Autodesk Inventor part; units mm, degrees
ref_plane "YZ Plane" through (0, 0, 0) normal (1, 0, 0) x (0, 1, 0)
ref_plane "XZ Plane" through (0, 0, 0) normal (0, 1, 0) x (-1, 0, 0)
ref_plane "XY Plane" through (0, 0, 0) normal (0, 0, 1) x (1, 0, 0)
sketch "草圖1" plane through (0, 0, 0) normal (0, 1, 0) x (-1, 0, 0)
  circle A0 centre (0, 0) radius 46.75
  circle A1 centre (0, 0) radius 44.75
  dimension "d0" = 93.5
  dimension "d1" = 2
extrude "擠出1" add sketch "草圖1" along normal blind 10
sketch "草圖2" plane through (0, 10, 0) normal (0, 1, 0) x (1, 0, 0)
  circle A0 centre (0, 0) radius 50
  dimension "d4" = 100
extrude "擠出2" add sketch "草圖2" along normal blind 2
sketch "草圖4" plane through (0, 0, 0) normal (1, 0, 0) x (0, 1, 0)
  line L0 (12, -50) -> (12, 50)
  line L1 (12, -25.0248) -> (30.0379, -25.0248)
  line L2 (30.0379, -25.0248) -> (30.0379, 11.7448)
  line L3 (30.0379, 11.7448) -> (12, 11.7448)
  line L4 (12, 11.7448) -> (12, -25.0248)
  line L5 (30.0379, -25.0248) -> (72.4644, 17.4017)
  line L6 (72.4644, 17.4017) -> (54.0796, 35.7864)
  line L7 (54.0796, 35.7864) -> (11.6532, -6.64)
  line L8 (11.6532, -6.64) -> (30.0379, -25.0248)
  point P0 (0, 0)
  dimension "d12" = 45
  dimension "d13" = 26
  dimension "d14" = 60
extrude "擠出4" add sketch "草圖4" along normal blind 5
fillet "圓角1" radius 10 1 edges at (2.5, 30.0379, 11.7448)
fillet "圓角2" radius 10 1 edges at (2.5, 30.0379, -25.0248)
sketch "草圖5" plane through (5, 0, 0) normal (1, 0, 0) x (0, 0, -1)
  line L0 (22.0958, 32.9669) -> (-17.4017, 72.4644)
  line L1 (-17.4017, 72.4644) -> (-35.7864, 54.0796)
  line L2 (-35.7864, 54.0796) -> (-14.6737, 32.9669)
  line L3 (20.7821, 30.0379) -> (-17.4017, 68.2217)
  line L4 (-17.4017, 68.2217) -> (-31.5438, 54.0796)
  line L5 (-31.5438, 54.0796) -> (-12.5524, 35.0882)
  line L6 (-31.5438, 54.0796) -> (-17.4017, 68.2217)
  line L7 (-17.4017, 68.2217) -> (20.7821, 30.0379)
  line L8 (20.7821, 30.0379) -> (6.64, 15.8958)
  line L9 (6.64, 15.8958) -> (-31.5438, 54.0796)
  arc A0 (25.0248, 25.8958) -> (22.0958, 32.9669) centre (15.0248, 25.8958) ccw
  line L10 (22.0958, 32.9669) -> (-17.4017, 72.4644)
  line L11 (-17.4017, 72.4644) -> (-35.7864, 54.0796)
  line L12 (-35.7864, 54.0796) -> (-14.6737, 32.9669)
  arc A1 (-11.7448, 25.8958) -> (-14.6737, 32.9669) centre (-21.7448, 25.8958) ccw
  line L13 (-11.7448, 25.8958) -> (-11.7448, 12)
  line L14 (25.0248, 12) -> (-11.7448, 12)
  line L15 (25.0248, 12) -> (25.0248, 25.8958)
  point P0 (0, 0)
  dimension "d19" = 20
  dimension "d20" = 54
  dimension "d21" = 54
extrude "擠出5" add sketch "草圖5" along normal blind 15
sketch "草圖6" plane through (0, 0, 0) normal (-1, 0, 0) x (0, 0, 1)
  circle A0 centre (12.4519, 49.1298) radius 10.5
  line L0 (12.4519, 49.1298) -> (26.594, 63.272)
  line L1 (17.4017, 72.4644) -> (35.7864, 54.0796)
  line L2 (-6.64, 15.8958) -> (-20.7821, 30.0379)
  point P0 (0, 0)
  dimension "d24" = 37
  dimension "d25" = 21
extrude "擠出6" cut sketch "草圖6" against normal blind 5
sketch "草圖7" plane through (5, 0, 0) normal (1, 0, 0) x (0, 0, -1)
  line L0 (-17.4017, 68.2217) -> (20.7821, 30.0379)
  line L1 (15.9031, 34.917) -> (20.7821, 30.0379)
  line L2 (20.7821, 30.0379) -> (15.1253, 24.3811)
  line L3 (15.1253, 24.3811) -> (10.2462, 29.2601)
  line L4 (10.2462, 29.2601) -> (15.9031, 34.917)
  point P0 (0, 0)
  dimension "d28" = 8
  dimension "d29" = 6.9
extrude "擠出7" add sketch "草圖7" along normal blind 13.8
sketch "草圖8" plane through (5, 0, 0) normal (1, 0, 0) x (0, 0, -1)
  line L0 (-17.2591, 39.7949) -> (6.64, 15.8958)
  line L1 (1.7609, 20.7749) -> (6.64, 15.8958)
  line L2 (6.64, 15.8958) -> (12.2968, 21.5527)
  line L3 (12.2968, 21.5527) -> (7.4178, 26.4317)
  line L4 (7.4178, 26.4317) -> (1.7609, 20.7749)
  point P0 (0, 0)
  dimension "d32" = 8
  dimension "d33" = 6.9
extrude "擠出8" add sketch "草圖8" along normal blind 13.8
sketch "草圖9" plane through (5, 0, 0) normal (1, 0, 0) x (0, 0, -1)
  line L0 (-17.4017, 68.2217) -> (20.7821, 30.0379)
  line L1 (-12.5226, 63.3427) -> (-17.4017, 68.2217)
  line L2 (-17.4017, 68.2217) -> (-23.0585, 62.5649)
  line L3 (-23.0585, 62.5649) -> (-18.1795, 57.6858)
  line L4 (-18.1795, 57.6858) -> (-12.5226, 63.3427)
  line L5 (6.64, 15.8958) -> (-31.5438, 54.0796)
  line L6 (-26.6648, 49.2005) -> (-31.5438, 54.0796)
  line L7 (-31.5438, 54.0796) -> (-25.8869, 59.7364)
  line L8 (-25.8869, 59.7364) -> (-21.0079, 54.8574)
  line L9 (-21.0079, 54.8574) -> (-26.6648, 49.2005)
  point P0 (0, 0)
  dimension "d36" = 8
  dimension "d37" = 8
  dimension "d38" = 6.9
extrude "擠出9" add sketch "草圖9" along normal blind 13.8
fillet "圓角3" radius 2 2 edges at (11.9, 54.8574, 21.0079) (11.9, 57.6858, 18.1795)
fillet "圓角4" radius 2 2 edges at (11.9, 26.4317, -7.4178) (11.9, 29.2601, -10.2462)
properties part number "第一關節"
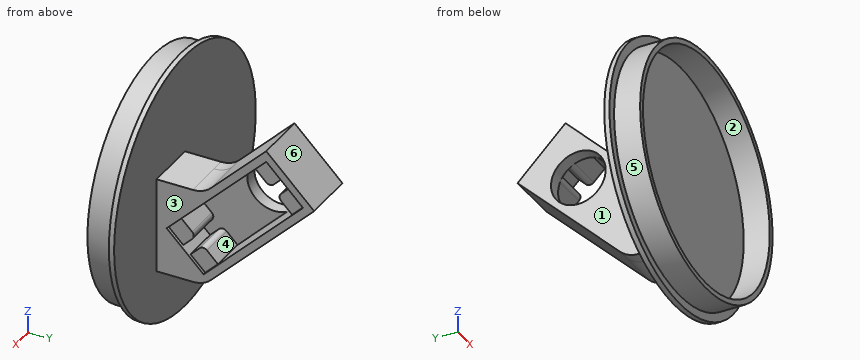
Can you work these out from the model? Positions are in its coordinate system, mm. Face numbers are marked on the shaded views. A direction names the side the tool comes from. Round coordinates to 2 decimals unless told otherwise and drop trailing zeros. Loops run counter-clockwise (first coordinate to the right, second up) from the corner with the lowest first, then second, coordinate; pieces in that order, holes last. Notation, with made-up numbers: M 60,60 L 101,60 A5 cw 101,68 Z; hole C 9,68.25 d11. An arc over 180 degrees is marked long. Write item = value, one per line. Start each with the question number.
(1) I need wall thicknesses on line 1 along Z through (x, y) = (0, 5); line 2 along Y through (x, z) = (16, -15); line 3 along X through (y, z) = (55, 23). Which ranges of each line are inside material? Lowest first, please.
(2) If we mould it in two halves opening along Y, with no side actions, what happens to the marked faces 4, 5 and 6? For each: released by +Y, released by -Y, zero draft, split by the parting line, or undercut.
(3) Suppose I cut it at B-B on y = 37. Write out the boundary of the cut face in (x, z).
(4) Suppose I cut it at A-A on z = 9.5. Write out the boundary of the cut face in (x, y).
(5) I'm going to push flat-ended pins straight in: P1, Ø5, axis at x = 2.5, z = -11.5, coming from the +Y side; P2, Ø8, axis at y = 21.5, z = -4.5, coming from the +X side; P3, Ø5, axis at y = 31.5, z = -15.5, coming from the +X side. Where does each tip first touch, or does it pass through?
(6) Suppose I cut it at C-C on x = 3.5. Write out the boundary of the cut face in (y, z).
(7) Suppose I cut it at D-D on z = 39.5. Write out the boundary of the cut face in (x, y).
(8) Which directions (+Z, -Z, +X, -X, +Y, -Y) give clear straight access to the entire face, cutting with the end or side of a thin tool? Please do the marked faces 1, 2 and 3.
Answer block:
q1.line_1 = -46.75 to -44.75, 44.75 to 46.75
q1.line_2 = 10 to 24.26, 24.51 to 34.01, 35.82 to 40.06
q1.line_3 = 0 to 18.8
q2.face_4 = undercut
q2.face_5 = zero draft
q2.face_6 = released by +Y
q3.outline = M 0,-18.06 L 20,-18.06 L 20,-13.82 L 5,-13.82 L 5,14.46 L 20,14.46 L 20,18.71 L 0,18.71 Z
q4.outline = M -49.09,10 L -45.77,10 L -45.77,0 L -43.73,0 L -43.73,10 L 43.73,10 L 43.73,0 L 45.77,0 L 45.77,10 L 49.09,10 L 49.09,12 L 20,12 L 20,32.04 L 5,32.04 L 5,39.05 L 0,39.05 L 0,12 L -49.09,12 Z; M 0,59.21 L 5,59.21 L 5,60.32 L 20,60.32 L 20,64.56 L 0,64.56 Z
q5.P1 = 46.06
q5.P2 = 20
q5.P3 = 18.8
q6.outline = M 0,-46.62 L 10,-46.62 L 10,-49.88 L 12,-49.88 L 12,-25.02 L 25.9,-25.02 A10 ccw 32.97,-22.1 L 72.46,17.4 L 54.08,35.79 L 32.97,14.67 A10 cw 25.9,11.74 L 12,11.74 L 12,49.88 L 10,49.88 L 10,46.62 L 0,46.62 L 0,44.61 L 10,44.61 L 10,-44.61 L 0,-44.61 Z; hole C 49.13,12.45 d21
q7.outline = M -30.66,10 L -25.01,10 L -25.01,0 L -21.03,0 L -21.03,10 L 21.03,10 L 21.03,0 L 25.01,0 L 25.01,10 L 30.66,10 L 30.66,12 L -30.66,12 Z
q8.face_1 = +Z, -Z, -X, +Y
q8.face_2 = -Y
q8.face_3 = +Z, -Z, +X, +Y
